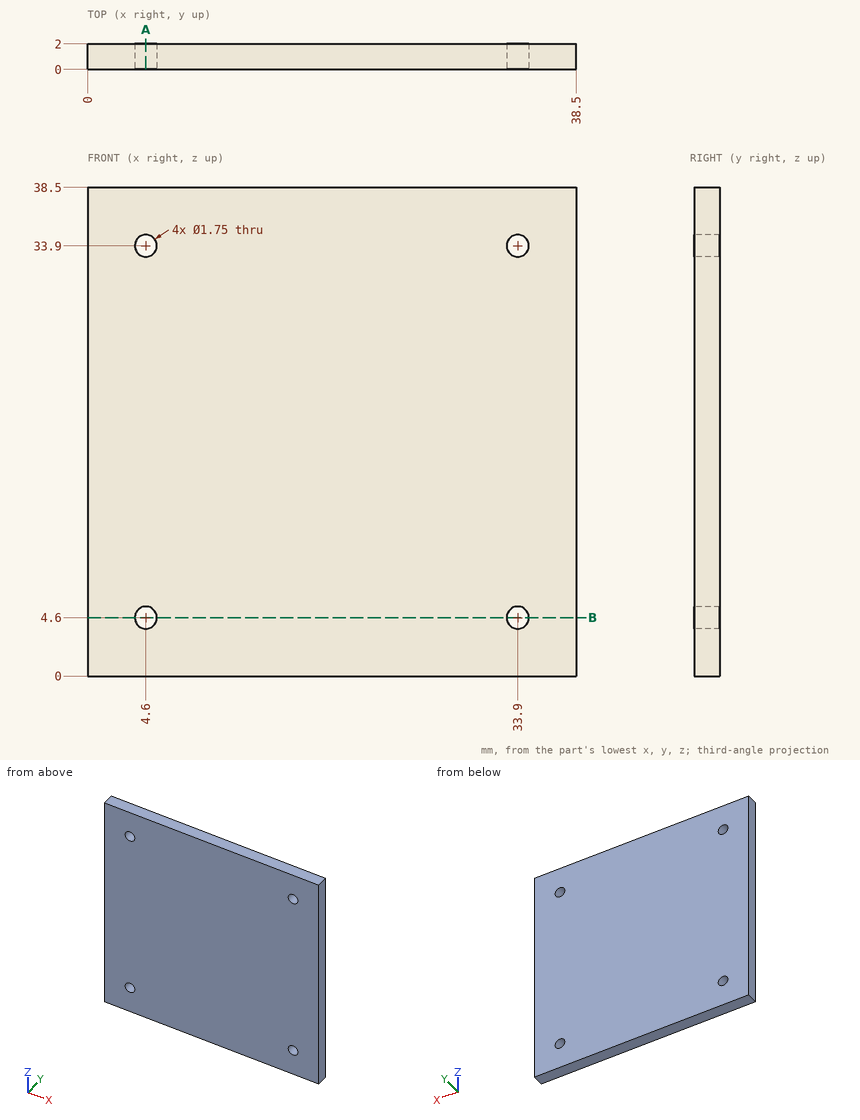
For this review, use the dimensioned drawing (mm, ordinates from the lowest corner) and the shaded views. Round coordinates to 2 decimals unless told otherwise and drop trailing zeros. Order: outer loops, then holes, each group sorted by start corner. A loop starts at its lowest first (then second) coordinate and runs counter-clockwise, first axis right, second up.
1) Consider section A-A (x = 4.6). State the section outline as (y, z) points (3 decimals).
The answers:
outline: (0, 0) - (2, 0) - (2, 3.725) - (0, 3.725) - close; (0, 5.475) - (2, 5.475) - (2, 33.025) - (0, 33.025) - close; (0, 34.775) - (2, 34.775) - (2, 38.5) - (0, 38.5) - close
2) Consider section B-B (z = 4.6). State the section outline as (x, y) points (3 decimals), plus the area to 3 significant figures.
The answers:
outline: (0, 0) - (3.725, 0) - (3.725, 2) - (0, 2) - close; (5.475, 0) - (33.025, 0) - (33.025, 2) - (5.475, 2) - close; (34.775, 0) - (38.5, 0) - (38.5, 2) - (34.775, 2) - close
area: 70.0 mm2
3) For L1, parallel to X at y = 1.6, z = 33.9 (3 decimals); L2, parallel to X at y = 1.85, z = 34.5, list the stretches that pass through material, from the lowest coordinate up.
The answers:
L1: x = 0 to 3.725, 5.475 to 33.025, 34.775 to 38.5
L2: x = 0 to 3.96, 5.24 to 33.26, 34.54 to 38.5
